from build123d import *

# Parameters (mm, degrees)
BOSS_EXTRUDE1_DEPTH             = 88.9
F_1_4_CLEARANCE_HOLE1_D         = 6.7564
CHAMFER1_SIZE                   = 12.7
SKETCH8_W                       = 69.85
SKETCH8_H                       = 177.8
BOSS_EXTRUDE4_DEPTH             = 6.35
SKETCH4_W                       = 177.8
SKETCH4_H                       = 19.05
BOSS_EXTRUDE2_DEPTH             = 2.38125
F_1_4_0_25_DIAMETER_HOLE1_D     = 6.35
F_1_4_0_25_DIAMETER_HOLE1_DEPTH = 11.938
F_1_4_0_25_DIAMETER_HOLE1_TIP   = 1.907732465
FILLET3_R                       = 12.7
BOSS_EXTRUDE7_DEPTH             = 34.925
SKETCH31_W                      = 16.271875
SKETCH31_H                      = 19.05
CUT_EXTRUDE1_DEPTH              = 186.839234959


with BuildPart() as part:
    # Sketch1 → Boss-Extrude1 (new, symmetric)
    with BuildSketch(Plane.XY):
        Polygon((-19.685, 22.225), (19.685, 22.225), (19.685, -15.875), (13.335, -15.875), (13.335, 15.875), (-13.335, 15.875), (-13.335, -15.875), (-19.685, -15.875), align=None)
    extrude(amount=BOSS_EXTRUDE1_DEPTH, both=True)

    # 1/4 Clearance Hole1 (through all)
    with Locations(Plane(origin=(19.685, 0, 0), x_dir=(0, 0, -1), z_dir=(1, 0, 0))):
        with Locations((-63.5, -9.525), (63.5, -9.525)):
            Hole(F_1_4_CLEARANCE_HOLE1_D / 2)

    # Chamfer1
    chamfer1_edges = [part.edges().sort_by_distance(p)[0] for p in [
        (16.51, -15.875, -88.9),
        (-16.51, -15.875, -88.9),
    ]]
    chamfer(chamfer1_edges, length=CHAMFER1_SIZE)

    # Sketch8 → Boss-Extrude4 (add)
    with BuildSketch(Plane(origin=(0, 22.225, 0), x_dir=(1, 0, 0), z_dir=(0, 1, 0))):
        Rectangle(SKETCH8_W, SKETCH8_H)
    extrude(amount=-BOSS_EXTRUDE4_DEPTH)

    # Sketch4 → Boss-Extrude2 (add, symmetric)
    with BuildSketch(Plane(origin=(0, 0, 0), x_dir=(0, 0, -1), z_dir=(1, 0, 0))):
        with Locations((0, 31.75)):
            Rectangle(SKETCH4_W, SKETCH4_H)
    extrude(amount=BOSS_EXTRUDE2_DEPTH, both=True)

    # 1/4 (0.25) Diameter Hole1
    with Locations(Plane.ZY.offset(2.38125)):
        with Locations((-76.2, 31.75), (76.2, 31.75), (54.428571429, 31.75), (32.657142857, 31.75), (10.885714286, 31.75), (-10.885714286, 31.75), (-32.657142857, 31.75), (-54.428571429, 31.75)):
            Hole(F_1_4_0_25_DIAMETER_HOLE1_D / 2, depth=F_1_4_0_25_DIAMETER_HOLE1_DEPTH)
            with Locations((0, 0, -(F_1_4_0_25_DIAMETER_HOLE1_DEPTH + F_1_4_0_25_DIAMETER_HOLE1_TIP / 2))):  # 118° drill point
                Cone(0, F_1_4_0_25_DIAMETER_HOLE1_D / 2, F_1_4_0_25_DIAMETER_HOLE1_TIP, mode=Mode.SUBTRACT)

    # Fillet3
    fillet3_edges = [part.edges().sort_by_distance(p)[0] for p in [
        (19.685, 15.875, 0),
        (-19.685, 15.875, 0),
    ]]
    fillet(fillet3_edges, radius=FILLET3_R)

    # Sketch30 → Boss-Extrude7 (add, symmetric)
    with BuildSketch(Plane(origin=(0, 0, 0), x_dir=(0, 0, -1), z_dir=(1, 0, 0))):
        Polygon((-88.9, 41.275), (-88.9, 27.481460305), (-87.337897471, 29.343101606), (-77.325845929, 41.275), align=None)
        Polygon((-59.089306097, 41.275), (-75.074154071, 22.225), (-71.539265332, 22.225), (-65.566468899, 29.343101606), (-55.554417358, 41.275), align=None)
        Polygon((-37.317877526, 41.275), (-53.3027255, 22.225), (-49.76783676, 22.225), (-43.795040328, 29.343101606), (-33.782988786, 41.275), align=None)
        Polygon((-12.011560215, 41.275), (-15.546448954, 41.275), (-31.531296928, 22.225), (-27.996408189, 22.225), (-22.023611756, 29.343101606), align=None)
        Polygon((9.759868357, 41.275), (6.224979617, 41.275), (-9.759868357, 22.225), (-6.224979617, 22.225), (-0.252183185, 29.343101606), align=None)
        Polygon((31.531296928, 41.275), (27.996408189, 41.275), (12.011560215, 22.225), (15.546448954, 22.225), (21.519245386, 29.343101606), align=None)
        Polygon((53.3027255, 41.275), (49.76783676, 41.275), (33.782988786, 22.225), (37.317877526, 22.225), (43.290673958, 29.343101606), align=None)
        Polygon((75.074154071, 41.275), (71.539265332, 41.275), (55.554417358, 22.225), (59.089306097, 22.225), (65.062102529, 29.343101606), align=None)
        Polygon((-88.9, 27.481460305), (-88.9, 22.225), (-78.854874309, 22.225), (-87.337897471, 29.343101606), align=None)
        Polygon((-65.566468899, 29.343101606), (-71.539265332, 22.225), (-57.083445738, 22.225), align=None)
        Polygon((-43.795040328, 29.343101606), (-49.76783676, 22.225), (-35.312017166, 22.225), align=None)
        Polygon((-22.023611756, 29.343101606), (-27.996408189, 22.225), (-13.540588595, 22.225), align=None)
        Polygon((8.230839976, 22.225), (-0.252183185, 29.343101606), (-6.224979617, 22.225), align=None)
        Polygon((30.002268548, 22.225), (21.519245386, 29.343101606), (15.546448954, 22.225), align=None)
        Polygon((51.773697119, 22.225), (43.290673958, 29.343101606), (37.317877526, 22.225), align=None)
        Polygon((73.545125691, 22.225), (65.062102529, 29.343101606), (59.089306097, 22.225), align=None)
        Polygon((88.9, 22.225), (88.9, 36.018539695), (77.325845929, 22.225), align=None)
    extrude(amount=BOSS_EXTRUDE7_DEPTH, both=True)

    # Sketch31 → Cut-Extrude1 (cut, through all)
    with BuildSketch(Plane.XY.offset(88.9)):
        with Locations((10.5171875, 31.75)):
            Rectangle(SKETCH31_W, SKETCH31_H)
        with Locations((-10.5171875, 31.75)):
            Rectangle(SKETCH31_W, SKETCH31_H)
    extrude(amount=-CUT_EXTRUDE1_DEPTH, mode=Mode.SUBTRACT)


solid = part.part
Geometry check sheet. Reference: the model listing, model coordinates, mm. A direction names the side the tool comes from. Coordinates: 2 decimals unless noted, no trailing zeros. Loops run counter-clockwise (first coordinate to the right, second up) from the corner with the lowest first, then second, coordinate; pieces in that order, holes last. Notation, with made-up numbers: (23.5, 16.25) - (44.5, 16.25) arc R16 cw to (44.5, 26.25) - close; hole circle Ø9 at (11, 84). An arc over 180 degrees is marked (long way). Use one line per item in the form item = value. Start each with the question number.
Item 1: Section check A-A, the plane y = 0. Enter the section's corners in (x, z) (3 decimals), and give its area (3 significant figures).
Item 2: Mould release check, pull along Y, two halves, no side actions. Record for faces 6 (the face through (-26.9, 35.23, -48.23)), 7 (the face through (-34.925, 23, 1)), 8 (the face through (17, -15.875, 8)), 9 (the face through (-26.9, 31.88, 23.43)): +Y half, -Y half, draft (parallel to the pull), parting line (faces both ways), or undercut.
Item 3: Section check C-C, the plane x = 10. Enter the section's corners in (y, z) (3 decimals).
Item 4: Section check B-B, the plane z = -16. Enter the section's corners in (x, y) (3 decimals), and give its area (3 significant figures).
Item 5: Section check D-D, the plane y = 7. Enter the section's corners in (x, z) (3 decimals).
Item 6: Thickness scan on probe 1 along X at (y, z) = (22.5, 50) (3 decimals); probe 2 along X at (y, z) = (-7.5, -58.5) (3 decimals); probe 3 along Y at (x, z) = (-15.75, 63.5) (3 decimals). Record the ranges inside material, lowest first.
Item 7: Tool access check on faces 1 (the face through (-26.9, 31.88, 1.66)), 2 (the face through (18.653, 29, -21)), 3 (the face through (26.675, 25.734, 83.037)), 4 (the face through (19.685, -6, 1)), 5 (the face through (-26.903, 25.734, -4.049)). Record the directions out of +Z, -Z, +X, -X, +Y, -Y that give a thin tool (end or side, any length) a straight path to the whole face; none if there is none.
Item 8: Gauge pin test, flat ends, axial feed: pin 1 (3 mm diameter, centred on x = -8, z = -42, fed in from +Y) (3 decimals); pin 2 (5 mm diameter, centred on x = 22.5, z = 63, fed in from +Y); pin 3 (7.5 mm diameter, centred on y = 31.75, z = 10.89, fed in from -X). Record the tip position at first contact, or that the pin passes through.
Computed:
q1.outline = (-19.685, -88.9) - (-13.335, -88.9) - (-13.335, 88.9) - (-19.685, 88.9) - close; (13.335, -88.9) - (19.685, -88.9) - (19.685, 88.9) - (13.335, 88.9) - close
q1.area = 2,260 mm2
q2.face_6 = undercut
q2.face_7 = draft
q2.face_8 = -Y half
q2.face_9 = +Y half
q3.outline = (15.875, -88.9) - (22.225, -88.9) - (22.225, 88.9) - (15.875, 88.9) - close
q4.outline = (-34.925, 15.875) - (-32.385, 15.875) arc R12.7 cw to (-19.685, 3.175) - (-19.685, -15.875) - (-13.335, -15.875) - (-13.335, 15.875) - (13.335, 15.875) - (13.335, -15.875) - (19.685, -15.875) - (19.685, 3.175) arc R12.7 cw to (32.385, 15.875) - (34.925, 15.875) - (34.925, 26.978) - (18.653, 26.978) - (18.653, 22.225) - (2.381, 22.225) - (2.381, 41.275) - (-2.381, 41.275) - (-2.381, 22.225) - (-18.653, 22.225) - (-18.653, 26.978) - (-34.925, 26.978) - close
q4.area = 1,160 mm2
q5.outline = (-20.275, -88.9) - (-13.335, -88.9) - (-13.335, 88.9) - (-20.275, 88.9) - close; (13.335, -88.9) - (20.275, -88.9) - (20.275, 88.9) - (13.335, 88.9) - close
q6.probe_1 = -34.925 to -18.653, -2.381 to 2.381, 18.653 to 34.925
q6.probe_2 = -19.685 to -13.335, 13.335 to 19.685
q6.probe_3 = -15.875 to -12.903, -6.147 to 22.225
q7.face_1 = -X, +Y
q7.face_2 = +Z, -Z, +Y
q7.face_3 = +X
q7.face_4 = +Z, -Z, +X, -Y
q7.face_5 = -X
q8.pin_1 = 22.225
q8.pin_2 = 39.59
q8.pin_3 = -2.38
